Check sheet for the modelled part. Datum: model origin and axes. Units: mm. A direction names the side the tool comes from. Give positions to 0.01 mm unless a question says otherwise; leave off trailing zeros. Order: outer loops, then holes, each group sorted by start corner. A loop starts at its lowest first (then second) coordinate and runs counter-clockwise, first axis right, second up.
```python
from build123d import *

# Parameters (mm, degrees)
F0_R     = 6.35
F1_DEPTH = 25.4
F2_R     = 4.445
F3_DEPTH = 17.78
F4_R     = 2.54


with BuildPart() as f1:
    # F0 (on Right) → F1 (new body)
    with BuildSketch(Plane.YZ):
        Circle(F0_R)
    extrude(amount=F1_DEPTH)

    # F2 (on face) → F3 (cut)
    with BuildSketch(Plane(origin=(0, 0, 0), x_dir=(0, -1, 0), z_dir=(-1, 0, 0))):
        Circle(F2_R)
    extrude(amount=-F3_DEPTH, mode=Mode.SUBTRACT)

    # F4
    f4_edges = [f1.edges().sort_by_distance(p)[0] for p in [
        (25.4, -6.35, 0),
    ]]
    fillet(f4_edges, radius=F4_R)


solid = f1.part
```
(1) Release check for a two-part mould opening along Y. For faces 3 (the face through (11.27, -1.38, -6.2)), 4 (the face through (25.4, 0, 0)), 5 (the face through (8.77, 0.96, -4.34)) record: released by +Y, released by -Y, zero draft, split by the parting line, or undercut.
(2) Go/stop test with flat-tipped pins: P1, Ø2, axis at x = 17, y = 0.5, coming from the -Z side; P2, Ø3, axis at x = 5.5, z = 3, coming from the -Y side; P3, Ø4, axis at x = 4, z = -2.5, coming from the +Y side; P4, Ø1, axis at x = 14.5, y = -5, coming from the +Z side. Record where each tip stops, or that it passes through.
(3) Thickness scan on L1, parallel to Z at x = 12.25, y = 0 (3 decimals); L2, parallel to X at y = -2.5, z = 0.75; L3, parallel to Y at x = 8.75, z = 1.75. Record the ranges inside material, lowest first.
(4) Tool access check on faces 1 (the face through (0, 3, -4)), 2 (the face through (17.78, 0, 0)). Record the directions out of +Z, -Z, +X, -X, +Y, -Y that give a thin tool (end or side, any length) a straight path to the whole face; none if there is none.
(5) Sectioned sample at A-A (z = 0). Enter the section's corners in (x, y) (3 decimals).
(6) Sectioned sample at C-C (x = 7.25). Enter the section's corners in (y, z) (3 decimals).
Values follow:
1. face 3: split by the parting line
1. face 4: zero draft
1. face 5: undercut
2. P1: stops at z = -6.35
2. P2: stops at y = -6.17
2. P3: stops at y = 6.33
2. P4: stops at z = 4.48
3. L1: z = -6.35 to -4.445, 4.445 to 6.35
3. L2: x = 17.78 to 25.4
3. L3: y = -6.1 to -4.09, 4.09 to 6.1
4. face 1: +Z, -Z, -X, +Y, -Y
4. face 2: -X
5. outline: (0, -6.35) - (22.86, -6.35) arc R2.54 ccw to (25.4, -3.81) - (25.4, 3.81) arc R2.54 ccw to (22.86, 6.35) - (0, 6.35) - (0, 4.445) - (17.78, 4.445) - (17.78, -4.445) - (0, -4.445) - close
6. outline: circle Ø12.7 at (0, 0); hole circle Ø8.89 at (0, 0)
